Source: CAD feature listing. Evaluate the final solid. Frame: model axes, mm. A direction names the side the tool comes from. Round coordinates to 2 decimals unless told otherwise and drop trailing zeros. Order: outer loops, then holes, each group sorted by start corner. A loop starts at its lowest first (then second) coordinate and runs counter-clockwise, first axis right, second up. Notation, with made-up numbers: (-26, 32) - (4, 32) arc R22 ccw to (4, 50) - close; hole circle Ø11 at (79.5, -35). An arc over 180 degrees is marked (long way). Return JSON: item names as keys, results as strings. Group by question number.
1) Section A-A, the plane y = 0. Return loops of the section in (x, z) (3 decimals).
2) Section D-D, the plane z = 10.79. Return loops of the section in (x, y) (1 decimal), plus the area to 3 significant figures.
3) Ray query, line 1 (Z direction, x = 31.75, y = 33); line 2 (Y direction, x = 10, z = 26) (3 decimals); line 3 (X direction, y = 18, z = 24) (3 decimals). Return the intervals inside material, ascending. Write a range as from..to.
4) Mould query, pull axis X, two halves, no side actions, for faces 5 (the cylindrical face through (-28.44, 21.46, 29.23)), 6 (the cylindrical face through (64.13, 31.275, 46.413)), 7 (the flat face through (-9, -19, 20.32)). Classes: pulls with the +X half, pulls with the -X half, needs draft (parallel to the pull), parting line crosses it, or undercut.
5) Section C-C, the plane y = 10.5. Return loops of the section in (x, z) (3 decimals), plus the area to 3 significant figures.
6) Contact query for flat-ended pins moving along their axis: P1, Ø3, axis at x = 47.625, y = 0, coming from the -Z side; P2, Ø3, axis at x = 52.5, y = -13.5, coming from the -Z side; P3, Ø3.5, axis at x = 15.75, z = 39.37, coming from the +Y side (3 decimals); P4, Ø1.5, axis at x = 7, z = 8.5, coming from the +Y side (3 decimals). Output: stop coordinate, or through.
7) Section B-B, the plane x = 15.75. Return loops of the section in (y, z) (3 decimals), plus the area to 3 significant figures.
8) Access query for faces 1 (the cylindrical face through (-36.19, 33.114, 26.115)), 2 (the flat face through (43.815, 0, 26)), 3 (the cylindrical face through (14.54, 31.375, 41.267)), 4 (the flat face through (16, -12.065, 6)). Directions: +Z, -Z, +X, -X, +Y, -Y. A direction counts if a zero-diameter tool reaches every point of the face in a straight line with its end or side. Return the directions, or none.
```python
from build123d import *

# Parameters (mm, degrees)
SKETCH1_W               = 114.3
SKETCH1_H               = 69.85
BOSS_EXTRUDE1_DEPTH     = 57.15
SKETCH2_W               = 114.3
SKETCH2_H               = 55.450000124
CUT_EXTRUDE2_DEPTH      = 25.4
SKETCH3_W               = 114.3
SKETCH3_H               = 46.99
CUT_EXTRUDE3_DEPTH      = 20.32
CUT_EXTRUDE6_REACH      = 108.824
SKETCH7_R               = 4.8
CUT_EXTRUDE7_DEPTH      = 75.121121315
CUT_EXTRUDE7_DEPTH_BACK = 75.121121315
SKETCH9_W               = 62.865
SKETCH9_H               = 55.450000124
SKETCH9_W_2             = 19.05
SKETCH9_H_2             = 69.85
CUT_EXTRUDE8_REACH      = 108.824
SKETCH8_R               = 2.25
SKETCH12_R              = 1.905
CUT_EXTRUDE10_DEPTH     = 19.05
SKETCH13_W              = 95.25
SKETCH13_H              = 8.925763794
CUT_EXTRUDE12_DEPTH     = 107.823534392
BOSS_EXTRUDE2_REACH     = 103.269
SKETCH14_W              = 20.32
SKETCH14_H              = 15.660000062
SKETCH5_R               = 2.415
CUT_EXTRUDE20_DEPTH     = 103.326545714
SKETCH18_W              = 20.32
SKETCH18_H              = 10.024904341
CUT_EXTRUDE21_DEPTH     = 113.329404355
BOSS_EXTRUDE4_DEPTH     = 8.89
F_8_CLEARANCE_HOLE1_D   = 4.4958
F_8_32_TAPPED_HOLE1_D   = 3.4544
SKETCH40_W              = 104.14
SKETCH40_H              = 12.835095659
CUT_EXTRUDE22_DEPTH     = 1.27
CUT_EXTRUDE24_DEPTH     = 108.544786288
FILLET3_R               = 6.35
CUT_EXTRUDE25_DEPTH     = 102.320780831
FILLET4_R               = 2.54


with BuildPart() as part:
    # Sketch1 → Boss-Extrude1 (new body)
    with BuildSketch(Plane.XY):
        Rectangle(SKETCH1_W, SKETCH1_H)
    extrude(amount=BOSS_EXTRUDE1_DEPTH)

    # Sketch2 → Cut-Extrude2 (cut)
    with BuildSketch(Plane.XY.offset(57.15)):
        Rectangle(SKETCH2_W, SKETCH2_H)
    extrude(amount=-CUT_EXTRUDE2_DEPTH, mode=Mode.SUBTRACT)

    # Sketch3 → Cut-Extrude3 (cut)
    with BuildSketch(Plane(origin=(0, 0, 0), x_dir=(-1, 0, 0), z_dir=(0, 0, -1))):
        with Locations((0, 11.43)):
            Rectangle(SKETCH3_W, SKETCH3_H)
    extrude(amount=-CUT_EXTRUDE3_DEPTH, mode=Mode.SUBTRACT)

    # Cut-Extrude6: up to this face of the body (flat: up to its plane)
    cut_extrude6_end = Plane(part.part.faces().sort_by_distance((0, 34.925, 38.735))[0])
    # Sketch7 → Cut-Extrude6 (cut, up to the picked face)
    with BuildSketch(Plane.XZ.offset(34.925), mode=Mode.PRIVATE) as cut_extrude6_sk1:
        with Locations((31.75, 39.37)):
            Circle(SKETCH7_R)
    cut_extrude6_tool1 = split(extrude(cut_extrude6_sk1.sketch, amount=-CUT_EXTRUDE6_REACH, mode=Mode.PRIVATE), bisect_by=cut_extrude6_end, keep=Keep.BOTH, mode=Mode.PRIVATE)
    add(cut_extrude6_tool1.solids().sort_by(Axis((31.75, -34.925, 39.37), (0, 1, 0)))[0], mode=Mode.SUBTRACT)

    # Sketch9 → Cut-Extrude7 (cut, two sides: drawn at the far end of the back side and taken through both)
    with BuildSketch(Plane.XY.offset(31.75).offset(-CUT_EXTRUDE7_DEPTH_BACK)):
        with Locations((12.3825, 0)):
            Rectangle(SKETCH9_W, SKETCH9_H)
        with Locations((-47.625, 0)):
            Rectangle(SKETCH9_W_2, SKETCH9_H_2)
    extrude(amount=CUT_EXTRUDE7_DEPTH + CUT_EXTRUDE7_DEPTH_BACK, mode=Mode.SUBTRACT)

    # Sketch8 → Cut-Extrude8 (cut, up to next)
    with BuildSketch(Plane(origin=(0, 34.925, 0), x_dir=(1, 0, 0), z_dir=(0, 1, 0)), mode=Mode.PRIVATE) as cut_extrude8_sk1:
        with Locations(Location((15.75, -39.37, 0), (0, 0, 180))):
            Circle(SKETCH8_R)
    cut_extrude8_tool1 = extrude(cut_extrude8_sk1.sketch, amount=-CUT_EXTRUDE8_REACH, mode=Mode.PRIVATE) & part.part
    # Sketch8 → Cut-Extrude8 (cut, up to next)
    with BuildSketch(Plane(origin=(0, 34.925, 0), x_dir=(1, 0, 0), z_dir=(0, 1, 0)), mode=Mode.PRIVATE) as cut_extrude8_sk2:
        with Locations(Location((47.75, -39.37, 0), (0, 0, 180))):
            Circle(SKETCH8_R)
    cut_extrude8_tool2 = extrude(cut_extrude8_sk2.sketch, amount=-CUT_EXTRUDE8_REACH, mode=Mode.PRIVATE) & part.part
    add(cut_extrude8_tool1.solids().sort_by_distance((15.75, 34.925, 39.37))[0], mode=Mode.SUBTRACT)
    add(cut_extrude8_tool2.solids().sort_by_distance((47.75, 34.925, 39.37))[0], mode=Mode.SUBTRACT)

    # Sketch12 → Cut-Extrude10 (cut)
    with BuildSketch(Plane(origin=(-19.05, 0, 0), x_dir=(0, 0, -1), z_dir=(1, 0, 0))):
        with Locations(Location((-27.94, -22.86, 0), (0, 0, 90))):
            Circle(SKETCH12_R)
        with Locations(Location((-27.94, 22.86, 0), (0, 0, 90))):
            Circle(SKETCH12_R)
    extrude(amount=-CUT_EXTRUDE10_DEPTH, mode=Mode.SUBTRACT)

    # Sketch13 → Cut-Extrude12 (cut, through all)
    with BuildSketch(Plane(origin=(0, 34.925, 0), x_dir=(1, 0, 0), z_dir=(0, 1, 0))):
        with Locations((9.525, -52.687118103)):
            Rectangle(SKETCH13_W, SKETCH13_H)
    extrude(amount=-CUT_EXTRUDE12_DEPTH, mode=Mode.SUBTRACT)

    # Sketch14 → Boss-Extrude2 (add, up to next)
    with BuildSketch(Plane.ZY.offset(-43.815), mode=Mode.PRIVATE) as boss_extrude2_sk1:
        with Locations((10.16, -19.895000031)):
            Rectangle(SKETCH14_W, SKETCH14_H)
    boss_extrude2_tool1 = extrude(boss_extrude2_sk1.sketch, amount=BOSS_EXTRUDE2_REACH, mode=Mode.PRIVATE) - part.part
    add(boss_extrude2_tool1.solids().sort_by_distance((43.815, -19.895, 10.16))[0])

    # Sketch5 → Cut-Extrude20 (cut, through all)
    with BuildSketch(Plane.XZ.offset(34.925)):
        with Locations((-3.81, 10.79)):
            Circle(SKETCH5_R)
        with Locations((46.99, 10.79)):
            Circle(SKETCH5_R)
    extrude(amount=-CUT_EXTRUDE20_DEPTH, mode=Mode.SUBTRACT)

    # Sketch18 → Cut-Extrude21 (cut, through all)
    with BuildSketch(Plane.ZY.offset(38.1)):
        with Locations((10.16, -29.91254783)):
            Rectangle(SKETCH18_W, SKETCH18_H)
    extrude(amount=-CUT_EXTRUDE21_DEPTH, mode=Mode.SUBTRACT)

    # Sketch26 → Boss-Extrude4 (add)
    with BuildSketch(Plane(origin=(57.15, 0, 0), x_dir=(0, 0, -1), z_dir=(1, 0, 0))):
        Polygon((-48.224236206, -34.925), (-20.32, -34.925), (-20.32, -24.900095659), (0, -24.900095659), (0, -12.065), (-20.32, -12.065), (-20.32, 34.925), (-48.224236206, 34.925), (-48.224236206, 27.725000062), (-31.75, 27.725000062), (-31.75, -27.725000062), (-48.224236206, -27.725000062), align=None)
    extrude(amount=BOSS_EXTRUDE4_DEPTH)

    # #8 Clearance Hole1 (through all)
    with Locations(Plane(origin=(0, 34.925, 0), x_dir=(1, 0, 0), z_dir=(0, 1, 0))):
        with Locations((59.69, -41.874236206)):
            Hole(F_8_CLEARANCE_HOLE1_D / 2)

    # #8-32 Tapped Hole1 (through all)
    with Locations(Plane.XY.offset(31.75)):
        with Locations((47.625, 0)):
            Hole(F_8_32_TAPPED_HOLE1_D / 2)

    # Sketch40 → Cut-Extrude22 (cut)
    with BuildSketch(Plane(origin=(0, 0, 0), x_dir=(-1, 0, 0), z_dir=(0, 0, -1))):
        with Locations((-13.97, -18.482547829)):
            Rectangle(SKETCH40_W, SKETCH40_H)
    extrude(amount=-CUT_EXTRUDE22_DEPTH, mode=Mode.SUBTRACT)

    # Sketch47 → Cut-Extrude24 (cut, through all)
    with BuildSketch(Plane(origin=(0, 34.925, 0), x_dir=(1, 0, 0), z_dir=(0, 1, 0))):
        Polygon((-38.1, -31.75), (-19.05, -31.75), (10.16, -48.224236206), (-38.1, -48.224236206), align=None)
    extrude(amount=-CUT_EXTRUDE24_DEPTH, mode=Mode.SUBTRACT)

    # Fillet3
    fillet3_edges = [part.edges().sort_by_distance(p)[0] for p in [
        (-38.1, -34.925, 26.035),
        (66.04, -31.325000031, 48.224236206),
        (66.04, 31.325000031, 48.224236206),
        (10.16, -31.325000031, 48.224236206),
        (10.16, 31.325000031, 48.224236206),
        (-19.05, -31.325000031, 31.75),
        (-19.05, 31.325000031, 31.75),
        (-38.1, 34.925, 26.035),
    ]]
    fillet(fillet3_edges, radius=FILLET3_R)

    # Sketch49 → Cut-Extrude25 (cut, through all)
    with BuildSketch(Plane.XZ.offset(24.900095659)):
        Polygon((-38.1, 20.32), (-32.302770819, 20.32), (-19.050248439, 1.27), (-38.1, 1.27), align=None)
        Polygon((1.32498508, 20.32), (10.16, 7.62), (33.02, 7.62), (43.815, 20.32), align=None)
        Polygon((66.04, 20.32), (49.8475, 1.27), (66.04, 1.27), align=None)
    extrude(amount=-CUT_EXTRUDE25_DEPTH, mode=Mode.SUBTRACT)

    # Fillet4
    fillet4_edges = [part.edges().sort_by_distance(p)[0] for p in [
        (15.398625781, -24.900095659, 1.27),
        (15.398625781, -12.065, 1.27),
        (49.8475, -18.48254783, 1.27),
        (1.32498508, -18.48254783, 20.32),
        (-19.050248439, -18.48254783, 1.27),
        (-32.302770819, -18.48254783, 20.32),
        (33.02, -18.48254783, 7.62),
    ]]
    fillet(fillet4_edges, radius=FILLET4_R)


solid = part.part
```
Geometry check:
{
 "1": {"outline": "(-38.1, 20.32) - (-19.05, 20.32) - (-19.05, 31.75) - (-38.1, 31.75) - close; (43.815, 20.32) - (45.898, 20.32) - (45.898, 31.75) - (43.815, 31.75) - close; (49.352, 20.32) - (66.04, 20.32) - (66.04, 31.75) - (49.352, 31.75) - close"},
 "2": {"outline": "(-25.7, -24.9) - (-6.2, -24.9) - (-6.2, -12.1) - (-25.7, -12.1) - close; (-1.4, -24.9) - (8, -24.9) - (8, -12.1) - (-1.4, -12.1) - close; (35.7, -24.9) - (44.6, -24.9) - (44.6, -12.1) - (35.7, -12.1) - close; (49.4, -24.9) - (57.9, -24.9) - (57.9, -12.1) - (49.4, -12.1) - close", "area": "593 mm2"},
 "3": {"line 1": "20.32..34.57, 44.17..48.22", "line 2": "-34.925..-27.725, 27.725..34.925", "line 3": "-38.1..-19.05, 43.815..66.04"},
 "4": {"face 5": "needs draft", "face 6": "pulls with the +X half", "face 7": "undercut"},
 "5": {"outline": "(-38.1, 20.32) - (-19.05, 20.32) - (-19.05, 31.75) - (-38.1, 31.75) - close; (43.815, 20.32) - (66.04, 20.32) - (66.04, 31.75) - (43.815, 31.75) - close", "area": "472 mm2"},
 "6": {"P1": "through", "P2": "z = 2.63", "P3": "y = -27.725", "P4": "y = -12.065"},
 "7": {"outline": "(-34.925, 20.32) - (-27.725, 20.32) - (-27.725, 48.224) - (-34.925, 48.224) - close; (-24.9, 3.81) arc R2.54 ccw to (-22.36, 1.27) - (-14.605, 1.27) arc R2.54 ccw to (-12.065, 3.81) - (-12.065, 7.62) - (-24.9, 7.62) - close; (27.725, 20.32) - (34.925, 20.32) - (34.925, 37.12) - (27.725, 37.12) - close; (27.725, 41.62) - (34.925, 41.62) - (34.925, 48.224) - (27.725, 48.224) - close", "area": "448 mm2"},
 "8": {"face 1": "+Z, -Z, -X, +Y", "face 2": "+Z", "face 3": "+Y", "face 4": "-Z, +X, -X, +Y"}
}
